Drawing for the job (mm, zero at the part's lowest x, y, z). Give positions to 0.01 mm unless a question says otherwise; leave off trailing zeros. Write each loop counter-clockwise with the first axis right and the second up, starting at its lowest first coordinate (ties: lowest second). Pieces come first, ordered by that corner, then holes.
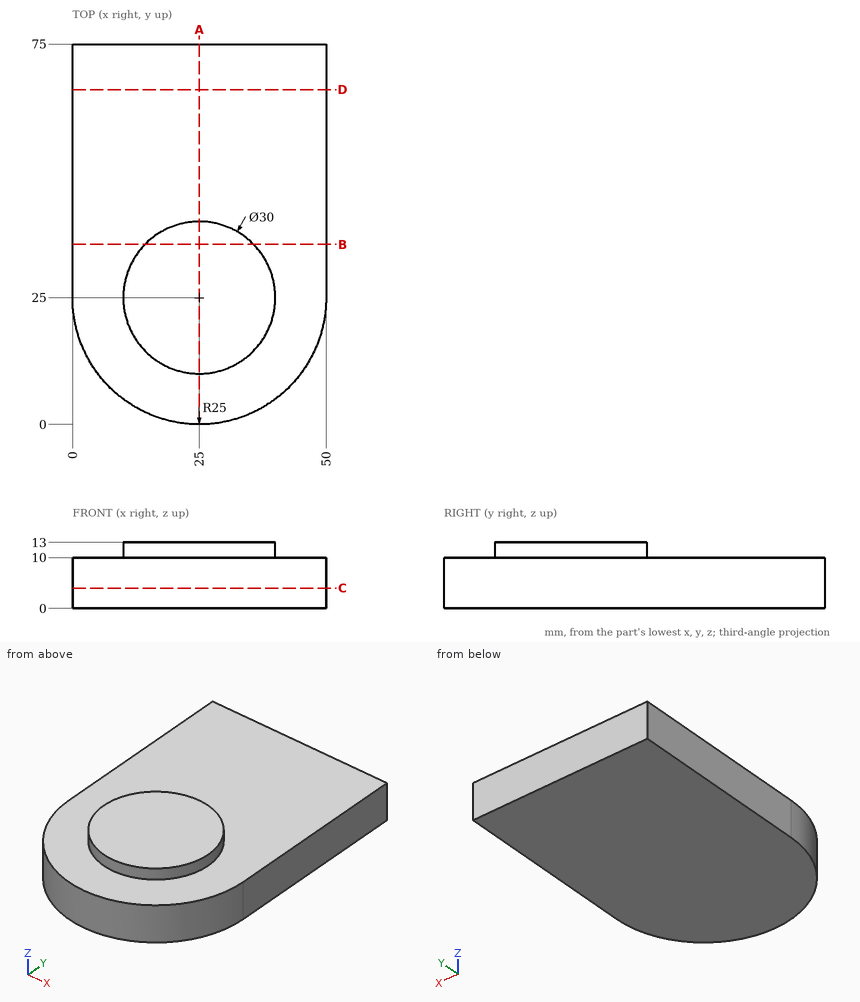
1. Slice it at A-A, the plane x = 25. Write the cut outline in (y, z), and give its area (3 significant figures).
Calculated:
outline: (0, 0) - (75, 0) - (75, 10) - (40, 10) - (40, 13) - (10, 13) - (10, 10) - (0, 10) - close
area: 840 mm2
2. Pin check, flat tips, straight feed: P1, Ø4, axis at x = 10, z = 3.5, coming from the -Y side; P2, Ø5, axis at x = 15, y = 59, coming from the -Z side. Stop position of each tip, or through.
Calculated:
P1: stops at y = 3.65
P2: stops at z = 0
3. Slice it at B-B, the plane y = 35.5. Write the cut outline in (x, z), and give its area (3 significant figures).
Calculated:
outline: (0, 0) - (50, 0) - (50, 10) - (35.71, 10) - (35.71, 13) - (14.29, 13) - (14.29, 10) - (0, 10) - close
area: 564 mm2
4. Slice it at D-D, the plane y = 66. Write the cut outline in (x, z).
Calculated:
outline: (0, 0) - (50, 0) - (50, 10) - (0, 10) - close
5. Slice it at C-C, the plane z = 4. Write the cut outline in (x, y).
Calculated:
outline: (0, 25) arc R25 ccw to (50, 25) - (50, 75) - (0, 75) - close
6. Probe probe 1 along Z at (x, y) = (5.5, 38); probe 2 along Y at (x, z) = (25, 3.5); probe 3 along X at (y, z) = (12.5, 9.75). List the from-to ranges inside material, lowest first.
Calculated:
probe 1: z = 0 to 10
probe 2: y = 0 to 75
probe 3: x = 3.35 to 46.65
